from build123d import *

# Parameters (mm, degrees)
F0_W     = 174
F0_H     = 20
F1_DEPTH = 13
F0_R     = 2.25
F2_DEPTH = 10
F0_W_2   = 5
F0_H_2   = 2
F3_DEPTH = 13


with BuildPart() as f1:
    # F0 (on Top) → F1 (new body)
    with BuildSketch(Plane.XY):
        with Locations((61.142166, 10)):
            Rectangle(F0_W, F0_H)
    extrude(amount=F1_DEPTH)

    # F0 (on Top) → F2 (join)
    with BuildSketch(Plane.XY):
        Polygon((-45.857834, 20), (-45.857834, 0), (-38.357834, 0), (-38.357834, 2), (-33.357834, 2), (-33.357834, 0), (-25.857834, 0), (-25.857834, 20), (-33.357834, 20), (-33.357834, 18), (-38.357834, 18), (-38.357834, 20), align=None)
        with Locations((-35.857834, 10)):
            Circle(F0_R, mode=Mode.SUBTRACT)
        Polygon((148.142166, 20), (148.142166, 0), (155.642166, 0), (155.642166, 2), (160.642166, 2), (160.642166, 0), (168.142166, 0), (168.142166, 20), (160.642166, 20), (160.642166, 18), (155.642166, 18), (155.642166, 20), align=None)
        with Locations((158.142166, 10)):
            Circle(F0_R, mode=Mode.SUBTRACT)
    extrude(amount=F2_DEPTH)

    # F0 (on Top) → F3 (join)
    with BuildSketch(Plane.XY):
        with Locations((-35.857834, 19)):
            Rectangle(F0_W_2, F0_H_2)
        with Locations((-35.857834, 1)):
            Rectangle(F0_W_2, F0_H_2)
        with Locations((158.142166, 19)):
            Rectangle(F0_W_2, F0_H_2)
        with Locations((158.142166, 1)):
            Rectangle(F0_W_2, F0_H_2)
    extrude(amount=F3_DEPTH)


solid = f1.part
Could you check a few things on this model? Use its own coordinates, in mm. Coordinates: 2 decimals unless noted, no trailing zeros. Write each loop counter-clockwise with the first axis right and the second up, starting at its lowest first coordinate (ties: lowest second). Pieces come first, ordered by that corner, then holes. Notation, with made-up numbers: (48.25, 1.5) - (66.25, 1.5) arc R12 ccw to (66.25, 20.5) - close; hole circle Ø7 at (75, -37). An arc over 180 degrees is marked (long way). Write item = value, one per line.
1) Will these pins go through, and if not, where does the flat tip stop? pin 1 Ø1 at (y, z) = (1.5, 11) entering from -X; pin 2 Ø1 at (y, z) = (19, 11) entering from +X; pin 3 Ø2.5 at (x, y) = (-35.86, 10) entering from +Z; pin 4 Ø0.9 at (y, z) = (6.5, 11) entering from +X.
Result set:
pin_1 = -38.36
pin_2 = 160.64
pin_3 = through
pin_4 = 148.14
2) We'd pull the mould along Y, two halves only. Please class faces 1 (the cylindrical face through (-33.712, 10.676, 4.93)), 2 (the flat face through (60, 0, 6)), 3 (the flat face through (60, 20, 6)), 4 (the flat face through (168.142, 10, 5)): +Y half, -Y half, draft (parallel to the pull), parting line (faces both ways), or undercut.
Result set:
face_1 = undercut
face_2 = -Y half
face_3 = +Y half
face_4 = draft
3) Suppose I cut it at A-A on y = 10. Please give me the cut outline in (x, z).
Result set:
outline = (-45.86, 0) - (-38.11, 0) - (-38.11, 10) - (-45.86, 10) - close; (-33.61, 0) - (155.89, 0) - (155.89, 10) - (148.14, 10) - (148.14, 13) - (-25.86, 13) - (-25.86, 10) - (-33.61, 10) - close; (160.39, 0) - (168.14, 0) - (168.14, 10) - (160.39, 10) - close
4) Please list where these lines run through material, in increasing order: line 1 (Y direction, x = -35.5, z = 3.75); line 2 (Z direction, x = 154.5, y = 2.5); line 3 (X direction, y = 6.75, z = 11.5). Write a range as [from, to].
Result set:
line_1 = [0, 7.78], [12.22, 20]
line_2 = [0, 10]
line_3 = [-25.86, 148.14]
